Verification items for this drawing (mm, ordinates from the low corner). Give positions to 0.01 mm unless a question says otherwise; leave off trailing zeros. Loops run counter-clockwise (first coordinate to the right, second up) from the corner with the lowest first, then second, coordinate; pieces in that order, holes last. Notation, with made-up numbers: (-5.5, -16) -> (19.5, -16) arc R22 ccw to (19.5, 0) -> close; hole circle Ø1 at (40, 12.5). An arc over 180 degrees is marked (long way). Write item = value, one per line.
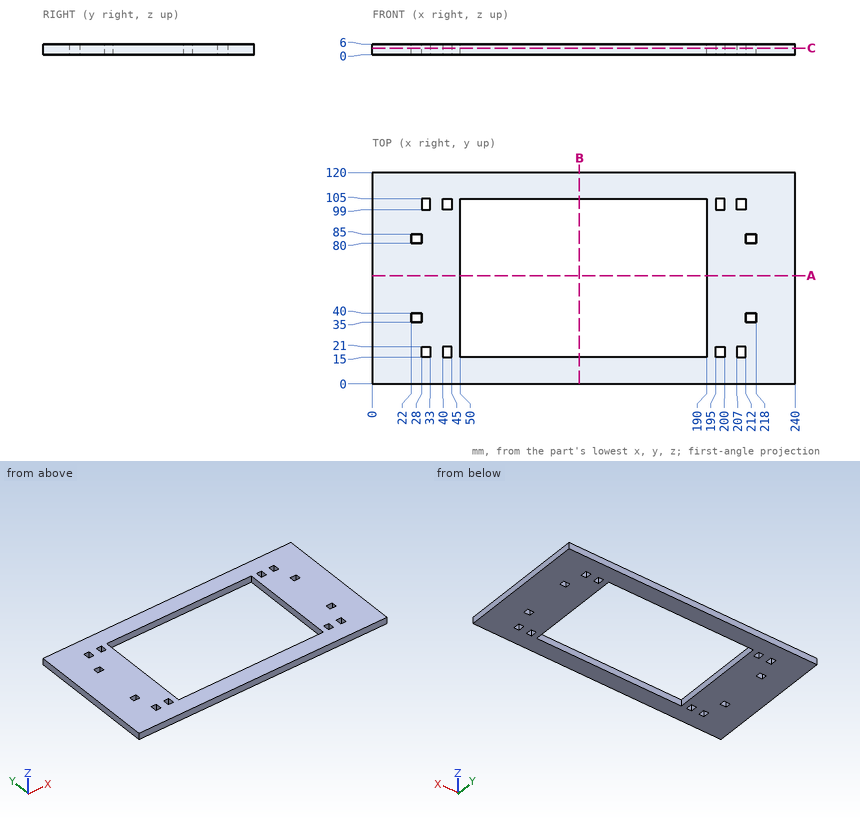
Item 1: Section check A-A, the plane y = 61.5. Record the cut outline in (x, z), plus the area to 3 significant figures.
Answer:
outline = (0, 0) -> (50, 0) -> (50, 6) -> (0, 6) -> close; (190, 0) -> (240, 0) -> (240, 6) -> (190, 6) -> close
area = 600 mm^2
Item 2: Thickness scan on L1, parallel to Y at x = 42.5, z = 5.15; L2, parallel to X at y = 102, z = 2.45; L3, parallel to X at y = 39.5, z = 1.35. Record the ranges inside material, lowest first. Write a range as [from, to].
Answer:
L1 = [0, 15], [21, 99], [105, 120]
L2 = [0, 28], [33, 40], [45, 50], [190, 195], [200, 207], [212, 240]
L3 = [0, 22], [28, 50], [190, 212], [218, 240]
Item 3: Section check B-B, the plane x = 117.5. Record the cut outline in (y, z).
Answer:
outline = (0, 0) -> (15, 0) -> (15, 6) -> (0, 6) -> close; (105, 0) -> (120, 0) -> (120, 6) -> (105, 6) -> close
Item 4: Section check C-C, the plane z = 3.6. Give the number of separate pieces and of enclosed holes in the cut face, plus the area to 3 significant figures.
Answer:
separate_pieces = 1
enclosed_holes = 13
area = 15,800 mm^2
